```python
from build123d import *

# Parameters (mm, degrees)
SKETCH_2_R               = 29.5
EXTRUDE_1_DEPTH          = 3
SKETCH_3_R               = 2
CUT_EXTRUDE_1_DEPTH      = 3
PATTERN_CIRCULAR_1_COUNT = 6
SKETCH_4_R               = 9
CUT_EXTRUDE_2_DEPTH      = 3
SKETCH_5_R               = 4
CUT_EXTRUDE_3_DEPTH      = 10


with BuildPart() as part:
    # 草图2 → 凸台-拉伸1 (new body)
    with BuildSketch(Plane.XY):
        Circle(SKETCH_2_R)
    extrude(amount=EXTRUDE_1_DEPTH)

    # 草图3 → 切除-拉伸1 (cut)
    with BuildSketch(Plane.XY.offset(3)):
        with Locations((-17.25, 0)):
            Circle(SKETCH_3_R)
    cut_extrude_1 = extrude(amount=-CUT_EXTRUDE_1_DEPTH, mode=Mode.SUBTRACT)

    # 阵列(圆周)1: 切除-拉伸1 ×6 about axis
    pattern_circular_1_axis = Axis((0.07965368, 0, 0), (0, 0, 1))
    for i in range(1, PATTERN_CIRCULAR_1_COUNT):
        add(cut_extrude_1.rotate(pattern_circular_1_axis, i * 360 / PATTERN_CIRCULAR_1_COUNT), mode=Mode.SUBTRACT)

    # 草图4 → 切除-拉伸2 (cut)
    with BuildSketch(Plane.XY.offset(3)):
        Circle(SKETCH_4_R)
    extrude(amount=-CUT_EXTRUDE_2_DEPTH, mode=Mode.SUBTRACT)

    # 草图5 → 切除-拉伸3 (cut)
    with BuildSketch(Plane.XY.offset(3)):
        with Locations((19.507246774, 11.74145424)):
            Circle(SKETCH_5_R)
    extrude(amount=-CUT_EXTRUDE_3_DEPTH, mode=Mode.SUBTRACT)


solid = part.part
```
For this review, take the finished solid that the model builds, in its own axes (mm). Coordinates: 2 decimals unless noted, no trailing zeros. Write each loop counter-clockwise with the first axis right and the second up, starting at its lowest first coordinate (ties: lowest second). Pieces come first, ordered by that corner, then holes. Notation, with made-up numbers: (57.5, 20) - (87.5, 20) arc R11 cw to (87.5, 40) - close; hole circle Ø8 at (-1.5, 44.5). An arc over 180 degrees is marked (long way). Answer in a Markdown table with one row per item. Add a question column.
Q1. Draft analysis for pull direction X (two halves, no side actions). For faces 1 (the cylindrical face through (-8.32, -16.99, 1.52)), 2 (the flat face through (-7, -6, 3)), 3 (the cylindrical face through (28.14, 8.86, 1.48)), state which applies: +X half, -X half, draft (parallel to the pull), parting line (faces both ways), or undercut.
Q2. For P1, Ø1.5, axis at x = 10.5, z = 2, coming from the -Y side, flat-tipped, find the tip position at first contact; note if it passes through.
Q3. We need section B-B, the plane y = 0. State the section outline as (x, z) points, and give its area (3 significant figures).
Q4. We need section D-D, the plane z = 1.25. Count the separate pieces of the cut face and the enclosed holes in it, and give its area (3 significant figures).
Q5. We need section C-C, the plane y = -14. State the section outline as (x, z) points.
Q6. For probe 1 along X at (y, z) = (15, 2.4); probe 2 along X at (y, z) = (14, 1.6); probe 3 along Y at (x, z) = (0, 2.2), list the stretches that pass through material, from the lowest coordinate up.
Q7. We need section A-A, the plane x = 0. State the section outline as (y, z) points, and give its area (3 significant figures).
Answer list:
| question | item | result |
|---|---|---|
| 1 | face 1 | undercut |
| 1 | face 2 | draft |
| 1 | face 3 | parting line |
| 2 | P1 | stops at y = -27.84 |
| 3 | outline | (-29.5, 0) - (-19.25, 0) - (-19.25, 3) - (-29.5, 3) - close; (-15.25, 0) - (-9, 0) - (-9, 3) - (-15.25, 3) - close; (9, 0) - (15.41, 0) - (15.41, 3) - (9, 3) - close; (19.41, 0) - (29.5, 0) - (29.5, 3) - (19.41, 3) - close |
| 3 | area | 99.0 mm2 |
| 4 | separate pieces | 1 |
| 4 | enclosed holes | 8 |
| 4 | area | 2,350 mm2 |
| 5 | outline | (-25.97, 0) - (-10.31, 0) - (-10.31, 3) - (-25.97, 3) - close; (-6.86, 0) - (7.02, 0) - (7.02, 3) - (-6.86, 3) - close; (10.47, 0) - (25.97, 0) - (25.97, 3) - (10.47, 3) - close |
| 6 | probe 1 | x = -25.4 to -10.59, -6.59 to 6.74, 10.74 to 17.19, 21.83 to 25.4 |
| 6 | probe 2 | x = -25.97 to -10.31, -6.86 to 7.02, 10.47 to 16.21, 22.81 to 25.97 |
| 6 | probe 3 | y = -29.5 to -9, 9 to 29.5 |
| 7 | outline | (-29.5, 0) - (-9, 0) - (-9, 3) - (-29.5, 3) - close; (9, 0) - (29.5, 0) - (29.5, 3) - (9, 3) - close |
| 7 | area | 123 mm2 |
